from build123d import *

# Parameters (mm, degrees)
ESQUISSE1_W             = 27.85
ESQUISSE1_H             = 200
BOSS_EXTRU_2_DEPTH      = 6
ENL_V_MAT_EXTRU_1_DEPTH = 6
ENL_V_START             = -3
ESQUISSE4_R             = 13.925
ENL_V_MAT_EXTRU_2_DEPTH = 3
ESQUISSE5_R             = 3
ENL_V_MAT_EXTRU_3_DEPTH = 3
ESQUISSE6_W             = 17.85
ESQUISSE6_H             = 23
ESQUISSE6_H_2           = 29
ENL_V_MAT_EXTRU_4_DEPTH = 10
CONG_1_R                = 10
CONG_2_R                = 10
ESQUISSE9_W             = 20.2
ESQUISSE9_H             = 40.3
ENL_V_MAT_EXTRU_7_DEPTH = 1.85


with BuildPart() as part:
    # Esquisse1 → Boss.-Extru.2 (new body)
    with BuildSketch(Plane.XY):
        with Locations((1.835077519, -78.788662791)):
            Rectangle(ESQUISSE1_W, ESQUISSE1_H)
        with BuildLine():
            Line((-12.089922481, 21.211337209), (15.760077519, 21.211337209))
            ThreePointArc((15.760077519, 21.211337209), (1.835077519, 35.136337209), (-12.089922481, 21.211337209))
        make_face()
    extrude(amount=BOSS_EXTRU_2_DEPTH)

    # Esquisse3 → Enlèv. mat.-Extru.1 (cut)
    with BuildSketch(Plane.XY.offset(6)):
        with BuildLine():
            Line((4.433153731, -172.288662791), (4.433153731, -169.288662791))
            ThreePointArc((4.433153731, -169.288662791), (-1.164922481, -170.788662791), (4.433153731, -172.288662791))
        make_face()
    extrude(amount=-ENL_V_MAT_EXTRU_1_DEPTH, mode=Mode.SUBTRACT)

    # Esquisse4 → Enlèv. mat.-Extru.2 (cut)
    with BuildSketch(Plane.XY.offset(6).offset(ENL_V_START)):
        with Locations((1.835077519, 21.211337209)):
            Circle(ESQUISSE4_R)
    extrude(amount=ENL_V_MAT_EXTRU_2_DEPTH, mode=Mode.SUBTRACT)

    # Esquisse5 → Enlèv. mat.-Extru.3 (cut)
    with BuildSketch(Plane.XY.offset(3)):
        with Locations((1.835077519, 21.211337209)):
            Circle(ESQUISSE5_R)
    extrude(amount=-ENL_V_MAT_EXTRU_3_DEPTH, mode=Mode.SUBTRACT)

    # Esquisse6 → Enlèv. mat.-Extru.4 (cut)
    with BuildSketch(Plane.XY.offset(6)):
        with BuildLine():
            Line((-7.089922481, -27.788662791), (10.760077519, -27.788662791))
            ThreePointArc((10.760077519, -27.788662791), (1.835077519, -18.863662791), (-7.089922481, -27.788662791))
        make_face()
        with Locations((1.835077519, -39.288662791)):
            Rectangle(ESQUISSE6_W, ESQUISSE6_H)
        with BuildLine():
            Line((-7.089922481, -50.788662791), (10.760077519, -50.788662791))
            ThreePointArc((10.760077519, -50.788662791), (1.835077519, -59.713662791), (-7.089922481, -50.788662791))
        make_face()
        with BuildLine():
            ThreePointArc((-7.089922481, -73.788662791), (1.835077519, -64.863662791), (10.760077519, -73.788662791))
            Line((10.760077519, -73.788662791), (-7.089922481, -73.788662791))
        make_face()
        with Locations((1.835077519, -88.288662791)):
            Rectangle(ESQUISSE6_W, ESQUISSE6_H_2)
        with BuildLine():
            Line((-7.089922481, -102.788662791), (10.760077519, -102.788662791))
            ThreePointArc((10.760077519, -102.788662791), (1.835077519, -111.713662791), (-7.089922481, -102.788662791))
        make_face()
        with BuildLine():
            Line((-7.089922481, -125.788662791), (10.760077519, -125.788662791))
            ThreePointArc((10.760077519, -125.788662791), (1.835077519, -116.863662791), (-7.089922481, -125.788662791))
        make_face()
        with Locations((1.835077519, -137.288662791)):
            Rectangle(ESQUISSE6_W, ESQUISSE6_H)
        with BuildLine():
            Line((-7.089922481, -148.788662791), (10.760077519, -148.788662791))
            ThreePointArc((10.760077519, -148.788662791), (1.835077519, -157.713662791), (-7.089922481, -148.788662791))
        make_face()
    extrude(amount=-ENL_V_MAT_EXTRU_4_DEPTH, mode=Mode.SUBTRACT)

    # Congé1
    cong_1_edges = [part.edges().sort_by_distance(p)[0] for p in [
        (-12.089922481, -178.788662791, 3),
    ]]
    fillet(cong_1_edges, radius=CONG_1_R)

    # Congé2
    cong_2_edges = [part.edges().sort_by_distance(p)[0] for p in [
        (15.760077519, -178.788662791, 3),
    ]]
    fillet(cong_2_edges, radius=CONG_2_R)

    # Esquisse9 → Enlèv. mat.-Extru.7 (cut)
    with BuildSketch(Plane(origin=(0, 0, 0), x_dir=(-1, 0, 0), z_dir=(0, 0, -1))):
        with Locations((-1.830077519, 10.911337209)):
            Rectangle(ESQUISSE9_W, ESQUISSE9_H)
    extrude(amount=-ENL_V_MAT_EXTRU_7_DEPTH, mode=Mode.SUBTRACT)


solid = part.part
The listing builds one solid part. Answer for the finished solid, in the listing's coordinates (mm). A direction names the side the tool comes from. Coordinates: 2 decimals unless noted, no trailing zeros. Loops run counter-clockwise (first coordinate to the right, second up) from the corner with the lowest first, then second, coordinate; pieces in that order, holes last.
1) Find section B-B on z = 5. Write down the section's boundary in (x, y) (3 decimals).
2) Determine the mould class of faces 4 (the face through (-12.09, -75, 3)), 5 (the face through (2.031, -18.866, 3.042)), 6 (the face through (-1.163, -170.679, 3.042)), 7 (the face through (11, -77, 6)) for opening direction X: pulls with the +X half, pulls with the -X half, needs draft (parallel to the pull), parting line crosses it, or undercut.
3) A tool of negligible diameter and unlimited length cuts with its end or side. For faces 1 (the face through (2.141, 35.133, 1.479)), 2 (the face through (2.03, -59.71, 3.04)), 3 (the face through (2, 25, 3)), from which of +Z, -Z, +X, -X, +Y, -Y can it reach the whole face along a straight path? Write none if from no direction.
4) Find section C-C on x = -5. Write down the section's boundary in (y, z).
5) Find section A-A on y = -34. Write down the section's boundary in (x, z).
6) Flat-ended cylindrical pins translate along their axes: pin 1 Ø3 at (x, z) = (8, 5.5) entering from -Y; pin 2 Ø2 at (x, z) = (4, 1) entering from +Y; pin 3 Ø10 at (x, y) = (-1.5, -44.5) entering from -Z; pin 4 Ø0.9 at (y, z) = (-170.5, 3) entering from -X. Find the tip coordinate at first contact, or state that the pin passes through.
7) Find the intervals of material crossed by L1, parallel to X at y = -101, z = 3.3; L2, parallel to Y at x = 6.75, z = 5.6; L3, parallel to Y at x = 3.25, z = 1.65, in increasing order.
Values:
1. outline: (-12.09, -168.789) arc R10 ccw to (-2.09, -178.789) - (5.76, -178.789) arc R10 ccw to (15.76, -168.789) - (15.76, 21.211) arc R13.925 cw to (-12.09, 21.211) - close; hole (-7.09, -148.789) arc R8.925 ccw to (10.76, -148.789) - (10.76, -125.789) arc R8.925 ccw to (-7.09, -125.789) - close; hole (-7.09, -102.789) arc R8.925 ccw to (10.76, -102.789) - (10.76, -73.789) arc R8.925 ccw to (-7.09, -73.789) - close; hole (-7.09, -50.789) arc R8.925 ccw to (10.76, -50.789) - (10.76, -27.789) arc R8.925 ccw to (-7.09, -27.789) - close; hole (4.433, -172.289) - (4.433, -169.289) arc R3 ccw (long way) to start
2. face 4: pulls with the -X half
2. face 5: undercut
2. face 6: undercut
2. face 7: needs draft
3. face 1: +Z, -Z, +Y
3. face 2: +Z, -Z
3. face 3: +Z, +Y
4. outline: (-178.36, 0) - (-154.53, 0) - (-154.53, 6) - (-178.36, 6) - close; (-120.05, 0) - (-108.53, 0) - (-108.53, 6) - (-120.05, 6) - close; (-68.05, 0) - (-56.53, 0) - (-56.53, 6) - (-68.05, 6) - close; (-22.05, 0) - (-9.24, 0) - (-9.24, 1.85) - (31.06, 1.85) - (31.06, 0) - (33.34, 0) - (33.34, 3) - (9.08, 3) - (9.08, 6) - (-22.05, 6) - close
5. outline: (-12.09, 0) - (-7.09, 0) - (-7.09, 6) - (-12.09, 6) - close; (10.76, 0) - (15.76, 0) - (15.76, 6) - (10.76, 6) - close
6. pin 1: stops at y = -178.76
6. pin 2: stops at y = 35.09
6. pin 3: passes through
6. pin 4: stops at x = -12.01
7. L1: x = -12.09 to -7.09, 10.76 to 15.76
7. L2: y = -178.74 to -156.24, -118.34 to -110.24, -66.34 to -58.24, -20.34 to 8.18
7. L3: y = -178.79 to -173.43, -168.14 to -157.6, -116.98 to -111.6, -64.98 to -59.6, -18.98 to -9.24, 31.06 to 35.06
